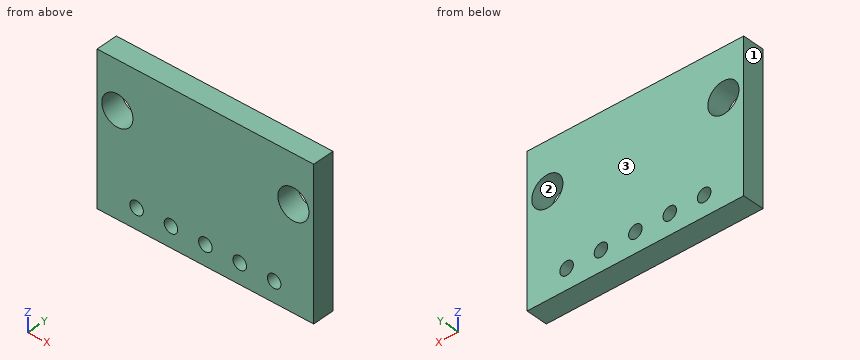
Autodesk Inventor part; units mm, degrees
ref_plane "YZ Plane" through (0, 0, 0) normal (1, 0, 0) x (0, 1, 0)
ref_plane "XZ Plane" through (0, 0, 0) normal (0, 1, 0) x (-1, 0, 0)
ref_plane "XY Plane" through (0, 0, 0) normal (0, 0, 1) x (1, 0, 0)
sketch "Sketch1" plane through (0, 0, 0) normal (0, 1, 0) x (-1, 0, 0)
  line L0 (-8, 5.5) -> (8, 5.5)
  line L1 (8, 5.5) -> (8, -5.5)
  line L2 (8, -5.5) -> (-8, -5.5)
  line L3 (-8, -5.5) -> (-8, 5.5)
  line L4 (-8, 5.5) -> (8, -5.5) construction
  line L5 (8, 5.5) -> (-8, -5.5) construction
  point P0 (0, 0)
  dimension "d0" = 16
  dimension "d1" = 11
extrude "Extrusion1" add sketch "Sketch1" along normal blind 1.6
sketch "Sketch2" plane through (0, 1.6, 0) normal (0, 1, 0) x (1, 0, 0)
  line L0 (8, -5.5) -> (8, 5.5)
  line L1 (-8, 5.5) -> (-8, -5.5)
  line L2 (8, 5.5) -> (-8, 5.5)
  point P0 (0, 0)
  point P1 (-6.5, -2)
  point P2 (6.5, -2)
  dimension "d4" = 1.5
  dimension "d5" = 1.5
  dimension "d6" = 7.5
  dimension "d7" = 7.5
hole "Hole1" at (-6.5, 1.6, 2) at (6.5, 1.6, 2) direction (0, -1, 0) diameter 2.3 end through all
sketch "Sketch3" plane through (0, 1.6, 0) normal (0, 1, 0) x (1, 0, 0)
  line L0 (-5.08, 4) -> (5.08, 4) construction
  line L1 (8, 5.5) -> (-8, 5.5)
  point P0 (0, 0)
  point P1 (0, 4)
  point P2 (-2.54, 4)
  point P3 (2.54, 4)
  point P4 (0, 4)
  dimension "d15" = 2.54
  dimension "d16" = 2.54
  dimension "d17" = 2.54
  dimension "d18" = 2.54
  dimension "d19" = 0
  dimension "d20" = 1.5
hole "Hole2" at (0, 1.6, -4) at (-2.54, 1.6, -4) at (-5.08, 1.6, -4) at (2.54, 1.6, -4) at (5.08, 1.6, -4) direction (0, -1, 0) diameter 1 end through all
properties part number "USB-C_BASE_plate"
The listing builds one solid part. Answer for the finished solid, in the listing's coordinates (mm). Face numbers are marked on the shaded views. Give positions to 0.01 mm unless a question says otherwise; leave off trailing zeros. Write each loop counter-clockwise with the first axis right and the second up, starting at its lowest first coordinate (ties: lowest second). Pieces come first, ordered by that corner, then holes. Notation, with made-up numbers: (-31, 87) -> (-1, 87) arc R5 cw to (-1, 96) -> close; hole circle Ø11 at (-3.75, -25.5). An arc over 180 degrees is marked (long way). Write item = value, one per line. Start each with the question number.
1) The part is cut by section C-C, the plane y = 0.25. Determine the outline of the cut face in (x, z).
2) Determine the mould class of the marked faces 1, 2 and 3 for opening direction X: +X half, -X half, draft (parallel to the pull), parting line (faces both ways), or undercut.
3) The part is cut by section B-B, the plane z = 2. Determine the outline of the cut face in (x, y).
4) The part is cut by section A-A, the plane x = -6.5. Determine the outline of the cut face in (y, z), and give its area (3 significant figures).
5) The part is cut by section D-D, the plane z = -4. Determine the outline of the cut face in (x, y).
6) Straight lines are drawn through the part: line 1 along X through (y, z) = (1.2, 2); line 2 along X through (y, z) = (0.85, -4); line 3 along Z through (x, y) = (-6.5, 0.4). For each, find the intervals that lie inside material, in ascending order.
7) This flat-tipped pin is pushed along its axis until it touches: pin 1 (4 mm diameter, centred on x = -6, z = 0.5, fed in from -Y). Where does it stop, or does it pass through?
Solutions:
q1.outline = (-8, -5.5) -> (8, -5.5) -> (8, 5.5) -> (-8, 5.5) -> close; hole circle Ø2.3 at (-6.5, 2); hole circle Ø1 at (-5.08, -4); hole circle Ø1 at (-2.54, -4); hole circle Ø1 at (0, -4); hole circle Ø1 at (2.54, -4); hole circle Ø1 at (5.08, -4); hole circle Ø2.3 at (6.5, 2)
q2.face_1 = -X half
q2.face_2 = undercut
q2.face_3 = draft
q3.outline = (-8, 0) -> (-7.65, 0) -> (-7.65, 1.6) -> (-8, 1.6) -> close; (-5.35, 0) -> (5.35, 0) -> (5.35, 1.6) -> (-5.35, 1.6) -> close; (7.65, 0) -> (8, 0) -> (8, 1.6) -> (7.65, 1.6) -> close
q4.outline = (0, -5.5) -> (1.6, -5.5) -> (1.6, 0.85) -> (0, 0.85) -> close; (0, 3.15) -> (1.6, 3.15) -> (1.6, 5.5) -> (0, 5.5) -> close
q4.area = 13.9 mm²
q5.outline = (-8, 0) -> (-5.58, 0) -> (-5.58, 1.6) -> (-8, 1.6) -> close; (-4.58, 0) -> (-3.04, 0) -> (-3.04, 1.6) -> (-4.58, 1.6) -> close; (-2.04, 0) -> (-0.5, 0) -> (-0.5, 1.6) -> (-2.04, 1.6) -> close; (0.5, 0) -> (2.04, 0) -> (2.04, 1.6) -> (0.5, 1.6) -> close; (3.04, 0) -> (4.58, 0) -> (4.58, 1.6) -> (3.04, 1.6) -> close; (5.58, 0) -> (8, 0) -> (8, 1.6) -> (5.58, 1.6) -> close
q6.line_1 = -8 to -7.65, -5.35 to 5.35, 7.65 to 8
q6.line_2 = -8 to -5.58, -4.58 to -3.04, -2.04 to -0.5, 0.5 to 2.04, 3.04 to 4.58, 5.58 to 8
q6.line_3 = -5.5 to 0.85, 3.15 to 5.5
q7.pin_1 = 0
